Autodesk Fusion 360 part; units mm, degrees
sketch "Sketch2" plane through (0, 0, 0) normal (0, 0, 1) x (-1, 0, 0)
  line L0 (29.6528, -57.1307) -> (30.0921, -57.0728)
  line L1 (30.0921, -57.0728) -> (30.5248, -56.9769)
  line L2 (30.5248, -56.9769) -> (30.9475, -56.8436)
  line L3 (30.9475, -56.8436) -> (31.3569, -56.674)
  line L4 (31.3569, -56.674) -> (31.75, -56.4694)
  line L5 (31.75, -56.4694) -> (32.1238, -56.2313)
  line L6 (32.1238, -56.2313) -> (32.4754, -55.9615)
  line L7 (32.4754, -55.9615) -> (32.8021, -55.6621)
  line L8 (32.8021, -55.6621) -> (33.1015, -55.3354)
  line L9 (33.1015, -55.3354) -> (33.3713, -54.9838)
  line L10 (33.3713, -54.9838) -> (33.6094, -54.61)
  line L11 (33.6094, -54.61) -> (33.814, -54.2169)
  line L12 (33.814, -54.2169) -> (33.9836, -53.8075)
  line L13 (33.9836, -53.8075) -> (34.1169, -53.3848)
  line L14 (34.1169, -53.3848) -> (34.2128, -52.9521)
  line L15 (34.2128, -52.9521) -> (34.2707, -52.5128)
  line L16 (34.2707, -52.5128) -> (34.29, -52.07)
  line L17 (34.29, -52.07) -> (34.29, 52.07)
  line L18 (34.29, 52.07) -> (34.2707, 52.5128)
  line L19 (34.2707, 52.5128) -> (34.2128, 52.9521)
  line L20 (34.2128, 52.9521) -> (34.1169, 53.3848)
  line L21 (34.1169, 53.3848) -> (33.9836, 53.8075)
  line L22 (33.9836, 53.8075) -> (33.814, 54.2169)
  line L23 (33.814, 54.2169) -> (33.6094, 54.61)
  line L24 (33.6094, 54.61) -> (33.3713, 54.9838)
  line L25 (33.3713, 54.9838) -> (33.1015, 55.3354)
  line L26 (33.1015, 55.3354) -> (32.8021, 55.6621)
  line L27 (32.8021, 55.6621) -> (32.4754, 55.9615)
  line L28 (32.4754, 55.9615) -> (32.1238, 56.2313)
  line L29 (32.1238, 56.2313) -> (31.75, 56.4694)
  line L30 (31.75, 56.4694) -> (31.3569, 56.674)
  line L31 (31.3569, 56.674) -> (30.9475, 56.8436)
  line L32 (30.9475, 56.8436) -> (30.5248, 56.9769)
  line L33 (30.5248, 56.9769) -> (30.0921, 57.0728)
  line L34 (30.0921, 57.0728) -> (29.6528, 57.1307)
  line L35 (29.6528, 57.1307) -> (29.21, 57.15)
  line L36 (29.21, 57.15) -> (-29.21, 57.15)
  line L37 (-29.21, 57.15) -> (-29.6528, 57.1307)
  line L38 (-29.6528, 57.1307) -> (-30.0921, 57.0728)
  line L39 (-30.0921, 57.0728) -> (-30.5248, 56.9769)
  line L40 (-30.5248, 56.9769) -> (-30.9475, 56.8436)
  line L41 (-30.9475, 56.8436) -> (-31.3569, 56.674)
  line L42 (-31.3569, 56.674) -> (-31.75, 56.4694)
  line L43 (-31.75, 56.4694) -> (-32.1238, 56.2313)
  line L44 (-32.1238, 56.2313) -> (-32.4754, 55.9615)
  line L45 (-32.4754, 55.9615) -> (-32.8021, 55.6621)
  line L46 (-32.8021, 55.6621) -> (-33.1015, 55.3354)
  line L47 (-33.1015, 55.3354) -> (-33.3713, 54.9838)
  line L48 (-33.3713, 54.9838) -> (-33.6094, 54.61)
  line L49 (-33.6094, 54.61) -> (-33.814, 54.2169)
  line L50 (-33.814, 54.2169) -> (-33.9836, 53.8075)
  line L51 (-33.9836, 53.8075) -> (-34.1169, 53.3848)
  line L52 (-34.1169, 53.3848) -> (-34.2128, 52.9521)
  line L53 (-34.2128, 52.9521) -> (-34.2707, 52.5128)
  line L54 (-34.2707, 52.5128) -> (-34.29, 52.07)
  line L55 (-34.29, 52.07) -> (-34.29, -52.07)
  line L56 (-34.29, -52.07) -> (-34.2707, -52.5128)
  line L57 (-34.2707, -52.5128) -> (-34.2128, -52.9521)
  line L58 (-34.2128, -52.9521) -> (-34.1169, -53.3848)
  line L59 (-34.1169, -53.3848) -> (-33.9836, -53.8075)
  line L60 (-33.9836, -53.8075) -> (-33.814, -54.2169)
  line L61 (-33.814, -54.2169) -> (-33.6094, -54.61)
  line L62 (-33.6094, -54.61) -> (-33.3713, -54.9838)
  line L63 (-33.3713, -54.9838) -> (-33.1015, -55.3354)
  line L64 (-33.1015, -55.3354) -> (-32.8021, -55.6621)
  line L65 (-32.8021, -55.6621) -> (-32.4754, -55.9615)
  line L66 (-32.4754, -55.9615) -> (-32.1238, -56.2313)
  line L67 (-32.1238, -56.2313) -> (-31.75, -56.4694)
  line L68 (-31.75, -56.4694) -> (-31.3569, -56.674)
  line L69 (-31.3569, -56.674) -> (-30.9475, -56.8436)
  line L70 (-30.9475, -56.8436) -> (-30.5248, -56.9769)
  line L71 (-30.5248, -56.9769) -> (-30.0921, -57.0728)
  line L72 (-30.0921, -57.0728) -> (-29.6528, -57.1307)
  line L73 (-29.6528, -57.1307) -> (-29.21, -57.15)
  line L74 (-29.21, -57.15) -> (29.21, -57.15)
  line L75 (29.21, -57.15) -> (29.6528, -57.1307)
  circle A0 centre (26.67, 50.025) radius 0.7
  circle A1 centre (20.32, 50.025) radius 0.7
  circle A2 centre (26.67, 33.795) radius 0.7
  circle A3 centre (20.32, 33.795) radius 0.7
  circle A4 centre (13.97, 50.025) radius 0.7
  circle A5 centre (13.97, 33.795) radius 0.7
  circle A6 centre (5.13, 26.87) radius 1.15
  circle A7 centre (29.21, 19.05) radius 1.75
  circle A8 centre (5.13, 22.17) radius 1.15
  circle A9 centre (5.13, 17.47) radius 1.15
  circle A10 centre (-0.1534, 50.7401) radius 1.75
  circle A11 centre (-14.15, 50.025) radius 0.7
  circle A12 centre (-0.17, 26.87) radius 1.15
  circle A13 centre (-5.47, 26.87) radius 1.15
  circle A14 centre (-14.15, 33.795) radius 0.7
  circle A15 centre (-20.5, 50.025) radius 0.7
  circle A16 centre (-26.85, 50.025) radius 0.7
  circle A17 centre (-20.5, 33.795) radius 0.7
  circle A18 centre (-26.85, 33.795) radius 0.7
  circle A19 centre (-0.17, 22.17) radius 1.15
  circle A20 centre (-5.47, 22.17) radius 1.15
  circle A21 centre (-0.17, 17.47) radius 1.15
  circle A22 centre (-5.47, 17.47) radius 1.15
  circle A23 centre (-0.17, 3.81) radius 0.45
  circle A24 centre (-0.17, 1.27) radius 0.45
  circle A25 centre (-29.21, 19.05) radius 1.75
  circle A26 centre (31.724, -24.1849) radius 0.45
  circle A27 centre (29.184, -24.1849) radius 0.45
  circle A28 centre (26.67, -36.505) radius 0.55
  circle A29 centre (24.13, -36.505) radius 0.55
  circle A30 centre (21.59, -36.505) radius 0.55
  circle A31 centre (29.21, -52.07) radius 1.75
  circle A32 centre (21.59, -44.45) radius 0.5
  circle A33 centre (19.05, -44.45) radius 0.5
  circle A34 centre (11.43, -44.45) radius 0.5
  circle A35 centre (8.89, -44.45) radius 0.5
  circle A36 centre (-13.105, -19.09) radius 0.4
  circle A37 centre (-17.985, -19.09) radius 0.4
  circle A38 centre (-0.205, -41.91) radius 0.5
  circle A39 centre (-2.745, -41.91) radius 0.5
  circle A40 centre (-5.285, -41.91) radius 0.5
  circle A41 centre (-29.21, -52.07) radius 1.75
  circle A42 centre (29.21, 19.05) radius 1.75
  circle A43 centre (-0.1534, 50.7401) radius 1.75
  circle A44 centre (-29.21, 19.05) radius 1.75
  circle A45 centre (29.21, -52.07) radius 1.75
  circle A46 centre (-29.21, -52.07) radius 1.75
  line L76 (-40.1186, 67.15) -> (39.8814, 67.15)
  line L77 (39.8814, 67.15) -> (39.8814, -72.85)
  line L78 (39.8814, -72.85) -> (-40.1186, -72.85)
  line L79 (-40.1186, -72.85) -> (-40.1186, 67.15)
  line L80 (-35.1186, -67.85) -> (-35.1186, 62.15)
  line L81 (-35.1186, 62.15) -> (34.8814, 62.15)
  line L82 (34.8814, 62.15) -> (34.8814, -67.85)
  line L83 (34.8814, -67.85) -> (-35.1186, -67.85)
  circle A47 centre (-35.1186, 62.15) radius 1.65
  circle A48 centre (34.8814, 62.15) radius 1.65
  circle A49 centre (34.8814, -67.85) radius 1.65
  circle A50 centre (-35.1186, -67.85) radius 1.65
  line L84 (-35.1186, 25.7548) -> (35.1185, 25.7548)
  line L85 (35.1185, 25.7548) -> (35.1185, 11.7548)
  line L86 (35.1185, 11.7548) -> (-35.1186, 11.7548)
  line L87 (-35.1186, 11.7548) -> (-35.1186, 25.7548)
  line L88 (-0.1186, 67.15) -> (-0.1186, -72.85) construction
  line L89 (-10.1186, 25.7548) -> (-10.1186, 11.7548)
  line L90 (9.8814, 25.7548) -> (9.8814, 11.7548)
  line L91 (-35.1186, -45.5115) -> (-22.1186, -45.5115)
  line L92 (-22.1186, -45.5115) -> (-22.1186, -58.5115)
  line L93 (-22.1186, -58.5115) -> (-35.1186, -58.5115)
  line L94 (-35.1186, -58.5115) -> (-35.1186, -45.5115)
  line L95 (21.8814, -45.5115) -> (21.8814, -58.5115)
  line L96 (34.8814, -45.5115) -> (21.8814, -45.5115)
  line L97 (21.8814, -58.5115) -> (34.8814, -58.5115)
  line L98 (-6.6186, 57.15) -> (6.3814, 57.15)
  line L99 (6.3814, 57.15) -> (6.3814, 44.15)
  line L100 (6.3814, 44.15) -> (-6.6186, 44.15)
  line L101 (-6.6186, 44.15) -> (-6.6186, 57.15)
  dimension "d1" = 80
  dimension "d2" = 140
  dimension "d4" = 5
  dimension "d6" = 3.3
  dimension "d7" = 3.3
  dimension "d8" = 3.3
  dimension "d9" = 3.3
  dimension "d11" = 14
  dimension "d12" = 10
  dimension "d13" = 13
  dimension "d14" = 13
  dimension "d15" = 13
  dimension "d16" = 13
  dimension "d35" = 10
extrude "Extrude1" add sketch "Sketch2" along normal blind 5 contours L0 L1 L2 L3 L4 L5 L6 L7 L8 L9 L10 L11 L12 L13 L14 L15 L16 L17 L74 L75 L95 L96 | L0 L1 L2 L3 L4 L5 L6 L7 L8 L9 L10 L11 L12 L13 L14 L15 L16 L17 L74 L75 L82 L95 L96 L97 | L74 L80 L82 L83 A49 A50 L92 L93 L95 L97 | L17 L55 L74 L86 L91 L92 L95 L96 | L55 L56 L57 L58 L59 L60 L61 L62 L63 L64 L65 L66 L67 L68 L69 L70 L71 L72 L73 L74 L80 L91 L92 L93 L94 | L55 L56 L57 L58 L59 L60 L61 L62 L63 L64 L65 L66 L67 L68 L69 L70 L71 L72 L73 L74 L91 L92 | L17 L82 L86 L96 | L55 L80 L86 L91 | L17 L84 L86 L90 | L17 L82 L84 L86 | L55 L80 L84 L86 L87 | L55 L84 L86 L89 | L17 L18 L19 L20 L21 L22 L23 L24 L25 L26 L27 L28 L29 L30 L31 L32 L33 L34 L35 L36 L37 L38 L39 L40 L41 L42 L43 L44 L45 L46 L47 L48 L49 L50 L51 L52 L53 L54 L55 A6 A12 A13 L84 L99 L100 L101 | L17 L18 L19 L20 L21 L22 L23 L24 L25 L26 L27 L28 L29 L30 L31 L32 L33 L34 L35 L36 L37 L38 L39 L40 L41 L42 L43 L44 L45 L46 L47 L48 L49 L50 L51 L52 L53 L54 L55 L80 L81 L82 A47 A48 L84 L98 | L82 L84 L85 L86 | A6 A12 A13 L84 L86 L89 L90 | A6 L84 | A6 L84 | A13 L84 | A13 L84 | A12 L84 | A12 L84 | L36 L98 L99 L100 L101 | A0 | A1 | A2 | A3 | A4 | A5 | A8 | A9 | A11 | A14 | A15 | A16 | A17 | A18 | A19 | A20 | A21 | A22 | A23 | A24 | A26 | A27 | A28 | A29 | A30 | A32 | A33 | A34 | A35 | A36 | A37 | A38 | A39 | A40 | L76 L77 L78 L79
extrude "Extrude2" add sketch "Sketch2" along normal blind 27 contours L0 L1 L2 L3 L4 L5 L6 L7 L8 L9 L10 L11 L12 L13 L14 L15 L16 L17 L74 L75 L95 L96 | L0 L1 L2 L3 L4 L5 L6 L7 L8 L9 L10 L11 L12 L13 L14 L15 L16 L17 L74 L75 L82 L95 L96 L97 | L55 L56 L57 L58 L59 L60 L61 L62 L63 L64 L65 L66 L67 L68 L69 L70 L71 L72 L73 L74 L80 L91 L92 L93 L94 | L55 L56 L57 L58 L59 L60 L61 L62 L63 L64 L65 L66 L67 L68 L69 L70 L71 L72 L73 L74 L91 L92 | L17 L84 L86 L90 | L17 L82 L84 L86 | L55 L80 L84 L86 L87 | L55 L84 L86 L89 | L82 L84 L85 L86 | L36 L98 L99 L100 L101
fillet "Fillet1" radius 3 2 edges at (-34.8814, 58.5115, 16) (35.1186, 58.5115, 16)
fillet "Fillet1" radius 3 6 edges at (35.1186, 45.5115, 16) (22.1186, 45.5115, 16) (22.1186, 58.5115, 16) (-21.8814, 45.5115, 16) (-21.8814, 58.5115, 16) (-34.8814, 45.5115, 16)
fillet "Fillet1" radius 3 4 edges at (6.6186, -44.15, 16) (6.6186, -57.15, 16) (-6.3814, -44.15, 16) (-6.3814, -57.15, 16)
fillet "Fillet2" radius 4 4 edges at (40.1186, 72.85, 2.5) (-39.8814, 72.85, 2.5) (40.1186, -67.15, 2.5) (-39.8814, -67.15, 2.5)
extrude "Extrude3" add sketch "Sketch2" along normal blind 20 contours A6 A12 A13 L84 L86 L89 L90 | A6 L84 | A13 L84 | A12 L84 | A8 | A9 | A19 | A20 | A21 | A22 picked at (5.0829, 25.7461) picked at (-5.5171, 25.7461) picked at (-0.2171, 25.7461)
fillet "Fillet3" radius 3 4 edges at (-9.8814, -18.7548, 20) (-9.8814, -18.7548, 27) (10.1186, -18.7548, 27) (10.1186, -18.7548, 20)
fillet "Fillet4" radius 3 4 edges at (35.1186, -25.7548, 16) (35.1186, -11.7548, 16) (-35.1185, -25.7548, 16) (-35.1185, -11.7548, 16)
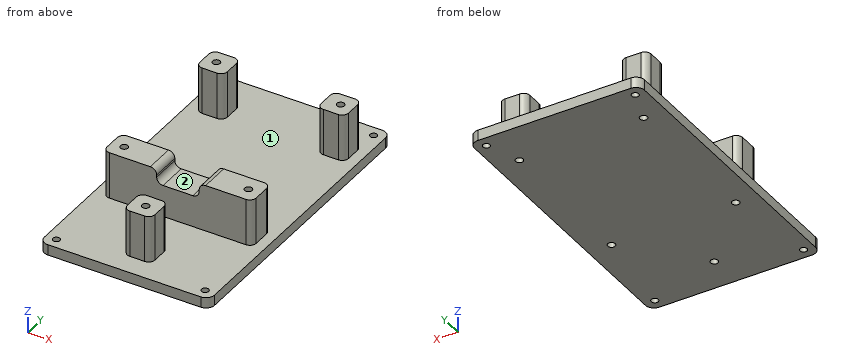
Source: CAD feature listing. Evaluate the final solid. Frame: model axes, mm. Face numbers are marked on the shaded views. Coordinates: 2 decimals unless noted, no trailing zeros. Loops run counter-clockwise (first coordinate to the right, second up) from the corner with the lowest first, then second, coordinate; pieces in that order, holes last. Notation, with made-up numbers: (-2, 32) - (54, 32) arc R20 cw to (54, 56) - close; hole circle Ø4 at (50, 79). An arc over 180 degrees is marked (long way). Return JSON: item names as keys, results as strings.
Q1. Mould query, pull axis Y, two halves, no side actions, for the marked faces 1 and 2. Classes: released by +Y, released by -Y, zero draft, split by the parting line, or undercut.
Results:
{"face 1": "undercut", "face 2": "zero draft"}
Q2. Section C-C, the plane z = 18.25. Give the number of separate pieces and of enclosed holes in the cut face, plus the area to 3 significant figures.
Results:
{"separate pieces": "4", "enclosed holes": "5", "area": "1,410 mm2"}
Q3. Section B-B, the plane x = -29.21. Return loops of the section in (y, z).
Results:
{"outline": "(-67.15, 0) - (-20.8, 0) - (-20.8, 27) - (-25.75, 27) - (-25.75, 5) - (-67.15, 5) - close; (-17.3, 0) - (50.32, 0) - (50.32, 27) - (45.51, 27) - (45.51, 5) - (-11.75, 5) - (-11.75, 27) - (-17.3, 27) - close; (53.82, 0) - (72.85, 0) - (72.85, 5) - (58.51, 5) - (58.51, 27) - (53.82, 27) - close"}
Q4. Section D-D, the plane y = -19.05. Return loops of the section in (x, z).
Results:
{"outline": "(-39.88, 0) - (-30.96, 0) - (-30.96, 27) - (-35.12, 27) - (-35.12, 5) - (-39.88, 5) - close; (-27.46, 0) - (27.46, 0) - (27.46, 27) - (13.12, 27) arc R3 ccw to (10.12, 24) - (10.12, 23) arc R3 cw to (7.12, 20) - (-6.88, 20) arc R3 cw to (-9.88, 23) - (-9.88, 24) arc R3 ccw to (-12.88, 27) - (-27.46, 27) - close; (30.96, 0) - (40.12, 0) - (40.12, 5) - (35.12, 5) - (35.12, 27) - (30.96, 27) - close"}
Q5. Material intervals for line 1 along X through (y, z) = (52.07, 13); line 2 along Y through (x, z) = (29.21, 21.5); line 3 along X through (y, z) = (-62.15, 2.75), sorted ascending.
Results:
{"line 1": "-34.88 to -30.96, -27.46 to -21.88, 22.12 to 27.46, 30.96 to 35.12", "line 2": "-25.75 to -20.8, -17.3 to -11.75, 45.51 to 50.32, 53.82 to 58.51", "line 3": "-39.88 to -36.53, -33.23 to 33.47, 36.77 to 40.12"}
Q6. Contact query for flat-ended pins moving along their axis: P1, Ø1, axis at x = 21.5, y = 2, coming from the +Z side; P2, Ø2, axis at y = -51.5, z = 16, coming from the +X side; P3, Ø4, axis at x = 0, y = -22, coming from the +Z side. Output: stop coordinate, or through.
Results:
{"P1": "z = 5", "P2": "x = 6.62", "P3": "z = 20"}
Q7. Section A-A, the plane y = 52.07. Return loops of the section in (x, z).
Results:
{"outline": "(-39.88, 0) - (-30.96, 0) - (-30.96, 27) - (-34.88, 27) - (-34.88, 5) - (-39.88, 5) - close; (-27.46, 0) - (27.46, 0) - (27.46, 27) - (22.12, 27) - (22.12, 5) - (-21.88, 5) - (-21.88, 27) - (-27.46, 27) - close; (30.96, 0) - (40.12, 0) - (40.12, 5) - (35.12, 5) - (35.12, 27) - (30.96, 27) - close"}
